from build123d import *

# Parameters (mm, degrees)
SKETCH_1_W          = 40
SKETCH_1_H          = 17
EXTRUDE_1_DEPTH     = 1.33
SKETCH_3_W          = 26
SKETCH_3_H          = 3.69
EXTRUDE_3_DEPTH     = 2
SKETCH_4_R          = 1.5
CUT_EXTRUDE_1_DEPTH = 22.823152843
SKETCH_2_W          = 4
SKETCH_2_H          = 6
EXTRUDE_4_DEPTH     = 10
SKETCH_5_W          = 5
SKETCH_5_H          = 6
EXTRUDE_5_DEPTH     = 4


with BuildPart() as part:
    # Эскиз1 → Бобышка-Вытянуть1 (new body)
    with BuildSketch(Plane(origin=(0, 0, 0), x_dir=(1, 0, 0), z_dir=(0, 1, 0))):
        Rectangle(SKETCH_1_W, SKETCH_1_H)
    extrude(amount=EXTRUDE_1_DEPTH)

    # Эскиз3 → Бобышка-Вытянуть3 (add)
    with BuildSketch(Plane.XZ):
        Polygon((-11, -8.5), (-6, -8.5), (-6, -0.19), (-6, 3.5), (-6, 8.5), (-11, 8.5), align=None)
        with Locations((7, 1.655)):
            Rectangle(SKETCH_3_W, SKETCH_3_H)
    extrude(amount=EXTRUDE_3_DEPTH)

    # Эскиз4 → Вырез-Вытянуть1 (cut, through all)
    with BuildSketch(Plane.XZ):
        with Locations(Location((16, -5.5, 0), (0, 0, 270))):
            Circle(SKETCH_4_R)
        with Locations(Location((-3, -5.5, 0), (0, 0, 270))):
            Circle(SKETCH_4_R)
    extrude(amount=-CUT_EXTRUDE_1_DEPTH, mode=Mode.SUBTRACT)

    # Эскиз2 → Бобышка-Вытянуть4 (add)
    with BuildSketch(Plane(origin=(0, 1.33, 0), x_dir=(1, 0, 0), z_dir=(0, 1, 0))):
        with Locations((12, 3.992967771)):
            Rectangle(SKETCH_2_W, SKETCH_2_H)
        with Locations((3, 3.992967771)):
            Rectangle(SKETCH_2_W, SKETCH_2_H)
    extrude(amount=EXTRUDE_4_DEPTH)

    # Эскиз5 → Бобышка-Вытянуть5 (add)
    with BuildSketch(Plane(origin=(0, 1.33, 0), x_dir=(1, 0, 0), z_dir=(0, 1, 0))):
        with Locations((7.5, 3.992967771)):
            Rectangle(SKETCH_5_W, SKETCH_5_H)
    extrude(amount=EXTRUDE_5_DEPTH)


solid = part.part
Work out the finished part from the listing and answer in its coordinate system (mm). A direction names the side the tool comes from. Round coordinates to 2 decimals unless told otherwise and drop trailing zeros. Order: outer loops, then holes, each group sorted by start corner. A loop starts at its lowest first (then second) coordinate and runs counter-clockwise, first axis right, second up. Notation, with made-up numbers: M 82,86.25 L 109,86.25 A26 ccw 109,110.25 Z; hole C 6.5,60 d2. An arc over 180 degrees is marked long. Put each result on its own line as item: value. Start each with the question number.
Q1. Straight lines are drawn through the part: L1, parallel to X at y = 0.6, z = -5.5; L2, parallel to X at y = 9.5, z = -4.25; L3, parallel to Y at x = 14.5, z = 1. For each, find the intervals that lie inside material, in ascending order. Write a range as [from, to].
Q2. Section B-B, the plane x = 16 is taken. Write down the section's boundary in (y, z).
Q3. Flat-ended cylindrical pins translate along their axes: pin 1 (3 mm diameter, centred on x = 1, y = 9, fed in from +Z); pin 2 (8.5 mm diameter, centred on x = -3.5, z = 0, fed in from +Y); pin 3 (1.8 mm diameter, centred on y = 7.5, z = -4, fed in from +X). Find the tip coordinate at first contact, or state that the pin passes through.
Q4. For a pull along X with two mould halves and no side action, classify faces 4 (the flat face through (10, 8, -4)), 5 (the flat face through (-11, -1, 0)), 6 (the flat face through (7, 0, -4)) as pulls with the +X half, pulls with the -X half, needs draft (parallel to the pull), parting line crosses it, or undercut.
Q5. Section D-D, the plane z = 6.75 is taken. Write down the section's boundary in (x, y), and give its area (3 significant figures).
Q6. Section A-A, the plane z = -5.5 is taken. Write down the section's boundary in (x, y).
Q7. A tool of negligible diameter and unlimited length cuts with its end or side. For faces 1 (the flat face through (7, 5, -0.993)), 2 (the flat face through (-6, -1, 6)), 3 (the flat face through (7, 5.33, -4)), from which of +Z, -Z, +X, -X, +Y, -Y can it reach the whole face along a straight path? Write none if from no direction.
Q8. Section C-C, the plane y = 0.75 is taken. Write down the section's boundary in (x, z).
Findings below:
1. L1: x = [-20, -4.5], [-1.5, 14.5], [17.5, 20]
1. L2: x = [1, 5], [10, 14]
1. L3: y = [-2, 1.33]
2. outline: M -2,-0.19 L 0,-0.19 L 0,-4 L 1.33,-4 L 1.33,8.5 L 0,8.5 L 0,3.5 L -2,3.5 Z; M 0,-8.5 L 1.33,-8.5 L 1.33,-7 L 0,-7 Z
3. pin 1: stops at z = -0.99
3. pin 2: stops at y = 1.33
3. pin 3: stops at x = 14
4. face 4: undercut
4. face 5: pulls with the -X half
4. face 6: needs draft
5. outline: M -20,0 L -11,0 L -11,-2 L -6,-2 L -6,0 L 20,0 L 20,1.33 L -20,1.33 Z
5. area: 63.2 mm^2
6. outline: M -20,0 L -11,0 L -11,-2 L -6,-2 L -6,0 L -4.5,0 L -4.5,1.33 L -20,1.33 Z; M -1.5,0 L 14.5,0 L 14.5,1.33 L 14,1.33 L 14,11.33 L 10,11.33 L 10,5.33 L 5,5.33 L 5,11.33 L 1,11.33 L 1,1.33 L -1.5,1.33 Z; M 17.5,0 L 20,0 L 20,1.33 L 17.5,1.33 Z
7. face 1: +Z, +X, -X, +Y
7. face 2: +Z, +X, -Y
7. face 3: +Z, -Z, +Y
8. outline: M -20,-8.5 L 20,-8.5 L 20,8.5 L -20,8.5 Z; hole C -3,-5.5 d3; hole C 16,-5.5 d3
